Here's the drawing with two shaded views (mm, measured from the low corner). I have some questions. A direction names the side the tool comes from. Coordinates: 2 decimals unless noted, no trailing zeros. Loops run counter-clockwise (first coordinate to the right, second up) from the corner with the lowest first, then second, coordinate; pieces in that order, holes last. Notation, with made-up numbers: M 84.5,10 L 120.5,10 A20 ccw 120.5,36 Z; hole C 38.25,87.25 d9. An arc over 180 degrees is marked long. Return JSON: item names as keys, results as strings. Group by question number.
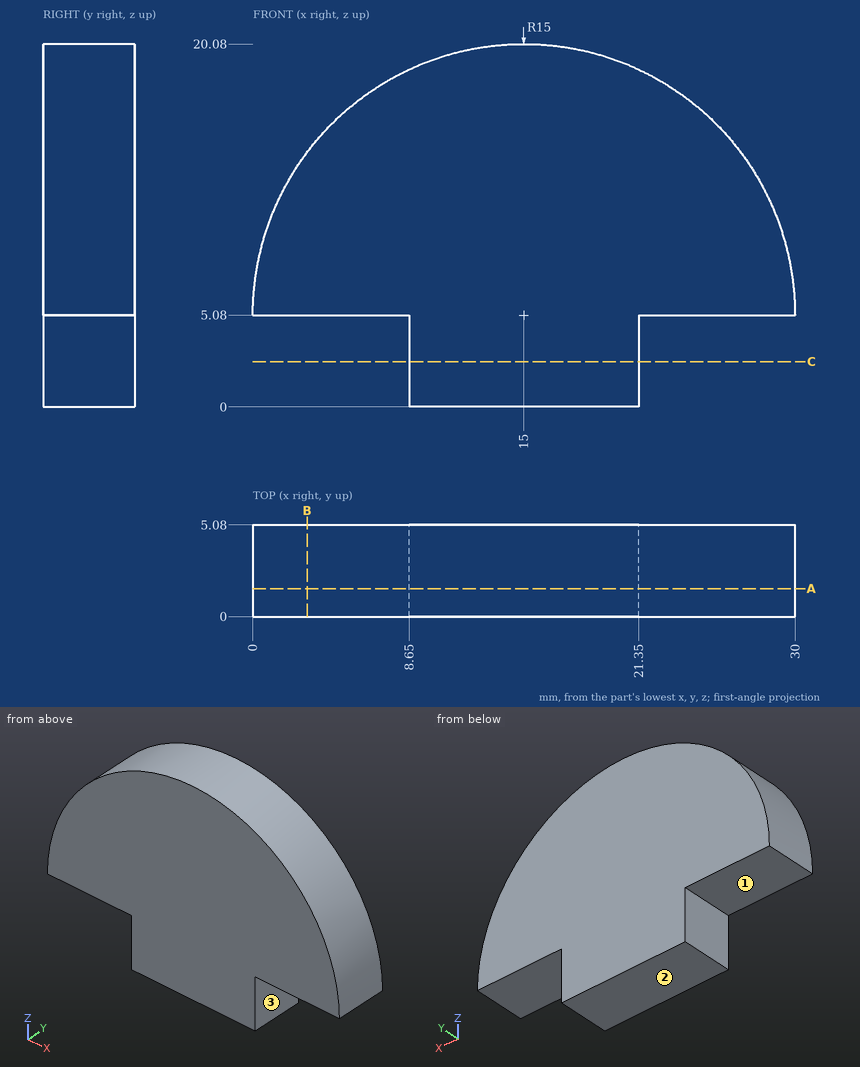
1) If I drill on line 1 (Z direction, x = 15.25, y = 2.1); line 2 (X direction, y = 3.65, z = 1.5); line 3 (X direction, y = 0.85, z = 17.5), over which ranges is the centre line in solid material (lowest first)? Write a range as from..to.
2) For the marked faces 1, 2 and 3, which set-ups out of +Z, -Z, +X, -X, +Y, -Y let a thin tool reach every point of the face, with its end or its side?
3) Suppose I cut it at A-A, the plane y = 1.55. List the corners of the cut face in (x, z) for me.
4) Suppose I cut it at C-C, the plane z = 2.5. List the corners of the cut face in (x, y) for me.
5) For pin 1 (2.5 mm diameter, centred on x = 24.5, y = 2.5, fed in from -Z); pin 2 (1 mm diameter, centred on x = 24, z = 3.5, fed in from -Y); pin 3 (2.5 mm diameter, centred on y = 1.5, z = 1.5, fed in from -X); pin 4 (1.5 mm diameter, centred on y = 2, z = 6.5, fed in from -X) (3 decimals), each with a flat end and sliding along its axis, tell me the tip position at first contact or that it passes through.
6) Suppose I cut it at B-B, the plane x = 3. List the corners of the cut face in (y, z) for me.
Returned:
{
 "1": {"line 1": "z = 0..20.08", "line 2": "x = 8.65..21.35", "line 3": "x = 6.59..23.41"},
 "2": {"face 1": "-Z, -X, +Y, -Y", "face 2": "-Z, +X, -X, +Y, -Y", "face 3": "-Z, +X, +Y, -Y"},
 "3": {"outline": "M 0,5.08 L 8.65,5.08 L 8.65,0 L 21.35,0 L 21.35,5.08 L 30,5.08 A15 ccw Z"},
 "4": {"outline": "M 8.65,0 L 21.35,0 L 21.35,5.08 L 8.65,5.08 Z"},
 "5": {"pin 1": "stops at z = 5.08", "pin 2": "passes through", "pin 3": "stops at x = 8.65", "pin 4": "stops at x = 0.015"},
 "6": {"outline": "M 0,5.08 L 5.08,5.08 L 5.08,14.08 L 0,14.08 Z"}
}
